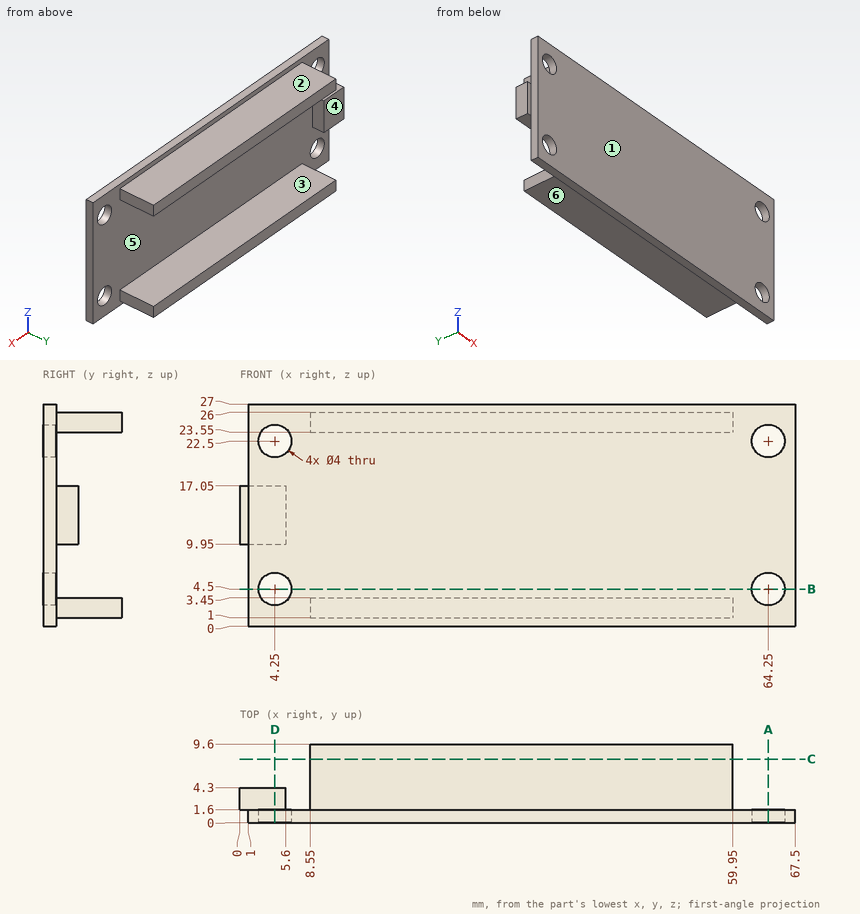
Study the drawing (mm; zero at the part's minimum x, y, z) and answer. A direction names the side the tool comes from. Round coordinates to 2 decimals unless told otherwise and drop trailing zeros. Write each loop counter-clockwise with the first axis right and the second up, starting at its lowest first coordinate (ties: lowest second). Pieces come first, ordered by that corner, then holes.
1) A cutting plane is placed at C-C on y = 7.75. Determine the outline of the cut face in (x, z), and give its area (3 significant figures).
2) Which of the six approach directions +Z, -Z, +X, -X, +Y, -Y give full straight-line access (tool end or side, diameter ignored) to the marked faces 1, 2 and 3?
3) A cutting plane is placed at A-A on x = 64.25. Determine the outline of the cut face in (y, z), and give its area (3 significant figures).
4) Consider probe 1 along X at (y, z) = (1.2, 22.5); probe 2 along Z at (x, y) = (64.25, 1); probe 3 along Z at (x, y) = (38, 9). Determine where each line is inside the solid, lowest interval first.
5) Determine the mould class of the marked faces 4, 5 and 6 for opening direction Z: pulls with the +Z half, pulls with the -Z half, needs draft (parallel to the pull), parting line crosses it, or undercut.
6) A cutting plane is placed at B-B on z = 4.5. Determine the outline of the cut face in (x, y), and give its area (3 significant figures).
7) A cutting plane is placed at D-D on x = 4.25. Determine the outline of the cut face in (y, z), and give its area (3 significant figures).
8) Flat-ended cylindrical pins translate along their axes: P1, Ø1.5, axis at y = 2, z = 18, coming from the -X side; P2, Ø1.4, axis at x = 3, y = 2.5, coming from the -Z side; P3, Ø2, axis at x = 35.5, z = 6.5, coming from the +Y side; P4, Ø1.5, axis at y = 5.5, z = 19.5, coming from the -X side. Find the tip coordinate at first contact, or state that the pin passes through.
Entries:
1. outline: (8.55, 1) - (59.95, 1) - (59.95, 3.45) - (8.55, 3.45) - close; (8.55, 23.55) - (59.95, 23.55) - (59.95, 26) - (8.55, 26) - close
1. area: 252 mm2
2. face 1: +Z, -Z, +X, -X, -Y
2. face 2: +Z, +X, -X, +Y
2. face 3: +X, -X, +Y
3. outline: (0, 0) - (1.6, 0) - (1.6, 2.5) - (0, 2.5) - close; (0, 6.5) - (1.6, 6.5) - (1.6, 20.5) - (0, 20.5) - close; (0, 24.5) - (1.6, 24.5) - (1.6, 27) - (0, 27) - close
3. area: 30.4 mm2
4. probe 1: x = 1 to 2.25, 6.25 to 62.25, 66.25 to 67.5
4. probe 2: z = 0 to 2.5, 6.5 to 20.5, 24.5 to 27
4. probe 3: z = 1 to 3.45, 23.55 to 26
5. face 4: needs draft
5. face 5: undercut
5. face 6: pulls with the -Z half
6. outline: (1, 0) - (2.25, 0) - (2.25, 1.6) - (1, 1.6) - close; (6.25, 0) - (62.25, 0) - (62.25, 1.6) - (6.25, 1.6) - close; (66.25, 0) - (67.5, 0) - (67.5, 1.6) - (66.25, 1.6) - close
6. area: 93.6 mm2
7. outline: (0, 0) - (1.6, 0) - (1.6, 2.5) - (0, 2.5) - close; (0, 6.5) - (1.6, 6.5) - (1.6, 9.95) - (4.3, 9.95) - (4.3, 17.05) - (1.6, 17.05) - (1.6, 20.5) - (0, 20.5) - close; (0, 24.5) - (1.6, 24.5) - (1.6, 27) - (0, 27) - close
7. area: 49.6 mm2
8. P1: stops at x = 1
8. P2: stops at z = 9.95
8. P3: stops at y = 1.6
8. P4: passes through
